Input: part model. Units: mm. Frame: model coordinates. Round coordinates to 2 decimals unless told otherwise and drop trailing zeros. Loops run counter-clockwise (first coordinate to the right, second up) from the corner with the lowest first, then second, coordinate; pieces in that order, holes last. Notation, with made-up numbers: M -13.5,27.5 L 35.5,27.5 A32 ccw 35.5,62.5 Z; hole C -33,-3 d3. An arc over 180 degrees is marked long. Put each result on its own line as item: value. Start each with the question number.
1) Line query: probe 1 along Z at (x, y) = (0.8, 87); probe 2 along Y at (x, z) = (0.15, -65.5); probe 3 along Y at (x, z) = (1.75, 62). Output: solid intervals per line, ascending.
2) Section A-A on z = 0. Output: boundary loops of the cut face in (x, y), plus the area to 3 significant figures.
3) Section D-D on y = -50.8. Output: boundary loops of the cut face in (x, z), plus the area to 3 significant figures.
4) Section C-C on x = 0.45. State how many separate pieces and enclosed holes the cut face has, plus the area to 3 significant figures.
5) Draft query along Y for faces 1 (the face through (0, 21, 1)), 2 (the face through (1.48, -19.53, -43.42)). Return one class per face: +Y half, -Y half, draft (parallel to the pull), parting line (faces both ways), or undercut.
6) Pin query (flat end, axial travel): pin 1 (14.5 mm diameter, centred on y = -22.51, z = -38.73, fed in from -X). Return the tip coordinate at first contact, or that it passes through.
7) Section B-B on y = 63.5. Output: boundary loops of the cut face in (x, z).
Autodesk Inventor part; units mm, degrees
ref_plane "Work Plane1" through (0, 0, 0) normal (1, 0, 0) x (0, 0, -1)
ref_plane "YZ Plane" through (0, 0, 0) normal (1, 0, 0) x (0, 1, 0)
ref_plane "XZ Plane" through (0, 0, 0) normal (0, 1, 0) x (-1, 0, 0)
sketch "Sketch1" plane through (0, 0, 0) normal (1, 0, 0) x (0, 1, 0)
  line L0 (101.6, 101.6) -> (101.6, -101.6)
  line L1 (101.6, -101.6) -> (-101.6, -101.6)
  line L2 (-101.6, -101.6) -> (-101.6, 101.6)
  line L3 (-101.6, 101.6) -> (101.6, 101.6)
  line L4 (-101.6, -101.6) -> (0, -101.6)
  circle A0 centre (63.5, 86.6) radius 3
  circle A1 centre (86.6, 63.5) radius 3
  circle A2 centre (63.5, -86.6) radius 3
  circle A3 centre (86.6, -63.5) radius 3
  circle A4 centre (-63.5, 86.6) radius 3
  circle A5 centre (-86.6, 63.5) radius 3
  circle A6 centre (-63.5, -86.6) radius 3
  circle A7 centre (-86.6, -63.5) radius 3
  circle A8 centre (-50.8, 0) radius 14.2875
  circle A9 centre (-9.965, 0) radius 11.1125
  circle A10 centre (-22.513, -38.7346) radius 5.5563
  circle A11 centre (-22.5126, 38.7346) radius 5.5563
  circle A12 centre (-47.9139, -38.7346) radius 5.5562
  circle A13 centre (2.8879, -38.7346) radius 5.5563
  circle A14 centre (2.8874, 38.7346) radius 5.5563
  circle A15 centre (-47.9126, 38.7346) radius 5.5563
  point P0 (0, 0)
  dimension "d28" = 28.575
  dimension "d30" = 22.225
  dimension "d39" = 6
  dimension "d42" = 38.1
  dimension "d43" = 38.1
  dimension "d44" = 38.1
  dimension "d45" = 38.1
  dimension "d46" = 15
  dimension "d47" = 38.1
  dimension "d49" = 15
  dimension "d50" = 15
  dimension "d51" = 15
  dimension "d52" = 38.1
  dimension "d53" = 15
  dimension "d57" = 101.6
  dimension "d58" = 50.8
  dimension "d60" = 40.835
  dimension "d61" = 203.2
  dimension "d62" = 203.2
  dimension "d63" = 101.6
  dimension "d64" = 101.6
  dimension "d65" = 91.635
  dimension "d66" = 38.1
  dimension "d67" = 38.1
  dimension "d68" = 15
  dimension "d69" = 15
  dimension "d70" = 15
  dimension "d71" = 101.6
  dimension "d72" = 101.6
  dimension "d91" = 11.1125
  dimension "d99" = 53.6861
  dimension "d100" = 25.4009
  dimension "d101" = 25.4009
ref_plane "Work Plane1" through (0, 0, 0) normal (1, 0, 0) x (0, 0, -1)
extrude "Extrusion4" add sketch "Sketch1" along normal blind 3
sketch "Sketch3" plane through (0, 0, 0) normal (-1, 0, 0) x (0, 0, 1)
  circle A0 centre (0, -50.8) radius 14.2875
  circle A1 centre (0, -9.965) radius 11.1125
  line L0 (101.6, -101.6) -> (-101.6, -101.6)
  line L1 (0, -50.8) -> (38.735, -50.8) construction
  line L2 (38.735, -50.8) -> (38.735, -69.112) construction
  circle A2 centre (38.735, -69.112) radius 2.5525
  line L3 (38.735, -69.112) -> (44.577, -69.112) construction
  circle A3 centre (44.577, -69.112) radius 2.0445
  line L4 (44.577, -69.112) -> (-44.577, -69.112) construction
  circle A4 centre (-44.577, -69.112) radius 2.0445
  line L5 (-44.577, -69.112) -> (-38.735, -69.112) construction
  circle A5 centre (-38.735, -69.112) radius 2.5525
  line L6 (0, -9.965) -> (37.592, -9.965) construction
  line L7 (37.592, -9.965) -> (37.592, 19.907) construction
  circle A6 centre (37.592, 19.907) radius 2.0445
  line L8 (37.592, 19.907) -> (31.75, 19.907) construction
  circle A7 centre (31.75, 19.907) radius 2.5525
  line L9 (37.592, 19.907) -> (-37.592, 19.907) construction
  circle A8 centre (-37.592, 19.907) radius 2.0445
  line L10 (-37.592, 19.907) -> (-31.75, 19.907) construction
  circle A9 centre (-31.75, 19.907) radius 2.5525
  point P0 (0, 0)
  dimension "d104" = 38.735
  dimension "d105" = 18.312
  dimension "d106" = 5.105
  dimension "d107" = 5.842
  dimension "d108" = 4.089
  dimension "d109" = 89.154
  dimension "d110" = 4.089
  dimension "d111" = 5.842
  dimension "d112" = 5.105
  dimension "d113" = 37.592
  dimension "d114" = 29.872
  dimension "d115" = 4.089
  dimension "d116" = 5.842
  dimension "d117" = 5.105
  dimension "d118" = 75.184
  dimension "d119" = 5.842
  dimension "d120" = 4.089
  dimension "d121" = 5.105
extrude "Extrusion5" cut sketch "Sketch3" against normal blind 10 contours A2 | A3 | A4 | A5 | A6 | A7 | A8 | A9
equation "\"d43\" = d42"
equation "\"d44\" = d43"
equation "\"d45\" = d42"
equation "\"d47\" = d44"
equation "\"d49\" = d46"
equation "\"d50\" = d46"
equation "\"d51\" = d50"
equation "\"d52\" = d42"
equation "\"d53\" = d51"
equation "\"d61\" = d62"
equation "\"d63\" = d57"
equation "\"d64\" = d63"
equation "\"d66\" = d43"
equation "\"d67\" = d47"
equation "\"d68\" = d50"
equation "\"d69\" = d68"
equation "\"d70\" = d53"
properties part number "Custom GearBox Mount"
Geometry results:
1. probe 1: z = -101.6 to -66.47, -60.53 to 60.53, 66.47 to 101.6
1. probe 2: y = -101.6 to -88.84, -84.36 to 84.36, 88.84 to 101.6
1. probe 3: y = -101.6 to -89.2, -84 to 84, 89.2 to 101.6
2. outline: M 0,-101.6 L 3,-101.6 L 3,-65.09 L 0,-65.09 Z; M 0,-36.51 L 3,-36.51 L 3,-21.08 L 0,-21.08 Z; M 0,1.15 L 3,1.15 L 3,101.6 L 0,101.6 Z
2. area: 457 mm²
3. outline: M 0,-101.6 L 3,-101.6 L 3,-43.48 L 0,-43.48 Z; M 0,-33.99 L 3,-33.99 L 3,-14.29 L 0,-14.29 Z; M 0,14.29 L 3,14.29 L 3,33.99 L 0,33.99 Z; M 0,43.48 L 3,43.48 L 3,101.6 L 0,101.6 Z
3. area: 467 mm²
4. separate pieces: 1
4. enclosed holes: 24
4. area: 39,300 mm²
5. face 1: draft
5. face 2: undercut
6. pin 1: stops at x = 0
7. outline: M 0,-101.6 L 3,-101.6 L 3,-89.6 L 0,-89.6 Z; M 0,-83.6 L 3,-83.6 L 3,83.6 L 0,83.6 Z; M 0,89.6 L 3,89.6 L 3,101.6 L 0,101.6 Z
